```python
from build123d import *

# Parameters (mm, degrees)
BOSS_EXTRUDE1_DEPTH = 3.175
SKETCH7_W           = 3.175
SKETCH7_H           = 8.89
CUT_EXTRUDE1_DEPTH  = 377.128183046


with BuildPart() as part:
    # Sketch3 → Boss-Extrude1 (new body)
    with BuildSketch(Plane.XY.offset(-652.571489798)):
        with BuildLine():
            Line((267.190410107, 14.374698747), (266.7, 14.276057895))
            Line((266.7, 14.276057895), (266.7, -23.769261632))
            add(Edge.make_bspline(
                [(266.7, -23.769261632), (275.880532182, -20.443051724), (285.029484636, -17.032239756), (303.244718304, -9.989758223), (312.307576038, -6.359638962), (330.31528392, 1.18765824), (339.262942891, 5.105981061), (356.976752757, 13.311628375), (365.744943517, 17.599570981), (374.396, 22.131936474)],
                knots=[0, 0, 0, 0, 0.25, 0.25, 0.5, 0.5, 0.75, 0.75, 1, 1, 1, 1], degree=3))
            Line((374.396, 22.131936474), (374.396, 35.91607659))
            add(Edge.make_bspline(
                [(374.396, 35.91607659), (360.350473035, 33.13205344), (346.312147582, 30.312088758), (318.38150515, 24.690232007), (304.489443265, 21.887076072), (290.596661876, 19.087501725)],
                knots=[0, 0, 0, 0, 0.5, 0.5, 0.994876875, 0.994876875, 0.994876875, 0.994876875], degree=3))
            ThreePointArc((290.596661876, 19.087501725), (281.24840199, 5.035600405), (267.190410107, 14.374698747))
        make_face()
    extrude(amount=BOSS_EXTRUDE1_DEPTH)

    # Sketch7 → Cut-Extrude1 (cut, through all)
    with BuildSketch(Plane.XY.offset(-649.396489798)):
        with Locations((320.548, 18.094665768)):
            Rectangle(SKETCH7_W, SKETCH7_H)
        with Locations((320.548, 4.124665768)):
            Rectangle(SKETCH7_W, SKETCH7_H)
    extrude(amount=-CUT_EXTRUDE1_DEPTH, mode=Mode.SUBTRACT)


solid = part.part
```
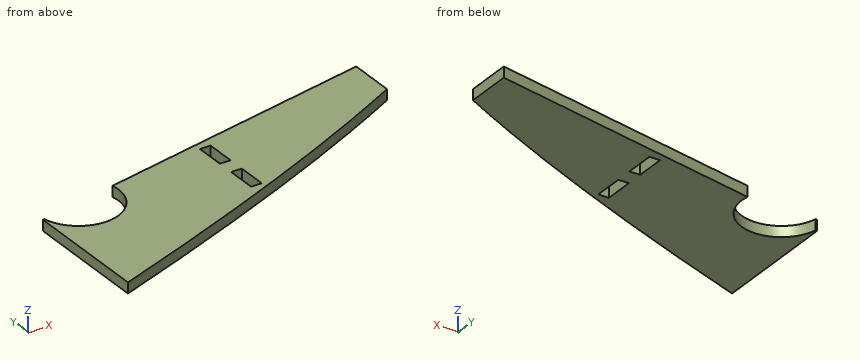
For this review, take the finished solid that the model builds, in its own axes (mm). Round coordinates to 2 decimals unless told otherwise and drop trailing zeros. Use a Markdown table: item, result.
Item 1: For pin 1 (1.6 mm diameter, centred on x = 320.5, z = -651, fed in from +Y), flat-tipped, find the tip position at first contact; note if it passes through.
Resolved:
| item | result |
|---|---|
| pin 1 | stops at y = 25.28 |
Item 2: For line 1 along X through (y, z) = (7, -652.25); line 2 along X through (y, z) = (7.5, -651.6); line 3 along X through (y, z) = (19, -651), list the stretches that pass through material, from the lowest coordinate up. Write a range as [from, to].
Resolved:
| item | result |
|---|---|
| line 1 | x = [266.7, 271.99], [285.8, 318.96], [322.14, 343.3] |
| line 2 | x = [266.7, 271.33], [286.45, 318.96], [322.14, 344.4] |
| line 3 | x = [290.61, 318.96], [322.14, 368.32] |
Item 3: Take a section at A-A (z = -651.2). State how many separate pieces and enclosed holes the cut face has, plus the area to 3 significant figures.
Resolved:
| item | result |
|---|---|
| separate pieces | 1 |
| enclosed holes | 2 |
| area | 2,660 mm² |
